Can you work these out from the model? Positions are in its coordinate system, mm. A direction names the side the tool comes from. Give positions to 0.01 mm unless a question says otherwise; leave off trailing zeros. Order: outer loops, then holes, each group sorted by start corner. A loop starts at its lowest first (then second) coordinate and runs counter-clockwise, first axis right, second up.
```python
from build123d import *

# Parameters (mm, degrees)
SKETCH1_W           = 23.3
SKETCH1_H           = 52.9
SKETCH1_W_2         = 19.3
SKETCH1_H_2         = 48.9
BOSS_EXTRUDE1_DEPTH = 47.4
SKETCH2_W           = 23.3
SKETCH2_H           = 52.9
BOSS_EXTRUDE2_DEPTH = 2
CUT_EXTRUDE1_DEPTH  = 2


with BuildPart() as part:
    # Sketch1 → Boss-Extrude1 (new body)
    with BuildSketch(Plane.XY):
        with Locations((9.65, 24.45)):
            Rectangle(SKETCH1_W, SKETCH1_H)
        with Locations((9.65, 24.45)):
            Rectangle(SKETCH1_W_2, SKETCH1_H_2, mode=Mode.SUBTRACT)
    extrude(amount=BOSS_EXTRUDE1_DEPTH)

    # Sketch2 → Boss-Extrude2 (add)
    with BuildSketch(Plane(origin=(0, 0, 0), x_dir=(-1, 0, 0), z_dir=(0, 0, -1))):
        with Locations((-9.65, 24.45)):
            Rectangle(SKETCH2_W, SKETCH2_H)
    extrude(amount=BOSS_EXTRUDE2_DEPTH)

    # Sketch3 → Cut-Extrude1 (cut)
    with BuildSketch(Plane.ZY.offset(2)):
        with BuildLine():
            Line((3, 44.7), (47.4, 44.7))
            ThreePointArc((47.4, 44.7), (51.4, 40.7), (47.4, 36.7))
            Line((47.4, 36.7), (3, 36.7))
            ThreePointArc((3, 36.7), (-1, 40.7), (3, 44.7))
        make_face()
    extrude(amount=-CUT_EXTRUDE1_DEPTH, mode=Mode.SUBTRACT)


solid = part.part
```
1) Suppose I cut it at B-B (z = 15). Please give me the cut outline in (x, y).
2) Suppose I cut it at C-C (x = 14). Please give me the cut outline in (y, z), and give its area (3 significant figures).
3) Which directions (+Z, -Z, +X, -X, +Y, -Y) give clear straight access to the entire face, cutting with the end or side of a thin tool? Please do faces 4 (the face through (10, 0, 23)), 5 (the face through (-1, 44.7, 25)), 6 (the face through (10, 25, -2)).
4) I'm going to push flat-ended pins straight in: pin 1 Ø3 at (x, y) = (12, 33.5) entering from +Z; pin 2 Ø8 at (x, y) = (15.5, 26) entering from +Z. Where does each tip first touch, or does it pass through?
5) We'd pull the mould along Y, two halves only. Please class faces 1 (the face through (-2, 24, 23)), 2 (the face through (10, 50.9, 23)), 3 (the face through (-1, 36.7, 26)): +Y half, -Y half, draft (parallel to the pull), parting line (faces both ways), or undercut.
6) If I drill on line 1 (Y direction, x = 5.5, z = 24); line 2 (X direction, y = 7.5, z = 13); line 3 (X direction, y = 38.5, z = 20.5), over which ranges is the centre line in solid material (lowest first)?
7) Suppose I cut it at A-A (y = 13). Please give me the cut outline in (x, z), and give its area (3 significant figures).
Results:
1. outline: (-2, -2) - (21.3, -2) - (21.3, 50.9) - (-2, 50.9) - (-2, 44.7) - (0, 44.7) - (0, 48.9) - (19.3, 48.9) - (19.3, 0) - (0, 0) - (0, 36.7) - (-2, 36.7) - close
2. outline: (-2, -2) - (50.9, -2) - (50.9, 47.4) - (48.9, 47.4) - (48.9, 0) - (0, 0) - (0, 47.4) - (-2, 47.4) - close
2. area: 295 mm2
3. face 4: +Z
3. face 5: +Z, -X
3. face 6: -Z, +X, -X, +Y, -Y
4. pin 1: stops at z = 0
4. pin 2: stops at z = 47.4
5. face 1: draft
5. face 2: +Y half
5. face 3: undercut
6. line 1: y = -2 to 0, 48.9 to 50.9
6. line 2: x = -2 to 0, 19.3 to 21.3
6. line 3: x = 19.3 to 21.3
7. outline: (-2, -2) - (21.3, -2) - (21.3, 47.4) - (19.3, 47.4) - (19.3, 0) - (0, 0) - (0, 47.4) - (-2, 47.4) - close
7. area: 236 mm2
